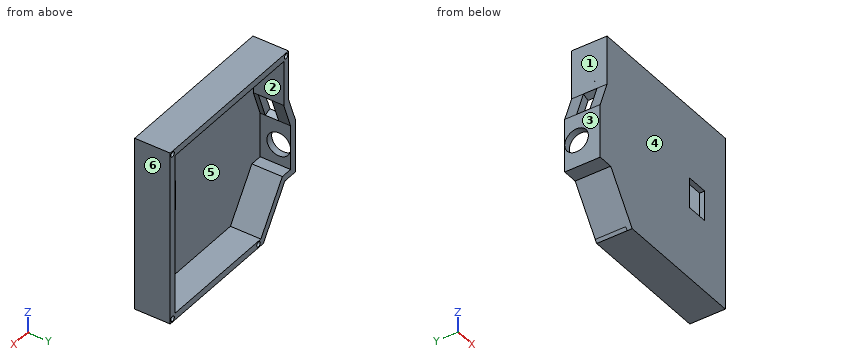
Autodesk Inventor part; units mm, degrees
ref_plane "YZ Plane" through (0, 0, 0) normal (1, 0, 0) x (0, 1, 0)
ref_plane "XZ Plane" through (0, 0, 0) normal (0, 1, 0) x (-1, 0, 0)
ref_plane "XY Plane" through (0, 0, 0) normal (0, 0, 1) x (1, 0, 0)
sketch "Sketch1" plane through (0, 0, 0) normal (0, 1, 0) x (-1, 0, 0)
  line L0 (0, 0) -> (49.1, 0)
  line L1 (49.1, -47.9) -> (0, -47.9)
  line L2 (0, -47.9) -> (0, 0)
  line L3 (46.7, -10.9) -> (49.1, -18.9)
  line L4 (46.7, -10.9) -> (46.7, 0)
  line L5 (49.1, 0) -> (46.7, 0)
  line L6 (49.1, -18.9) -> (49.1, -47.9)
  dimension "d0" = 49.1
  dimension "d1" = 47.9
  dimension "d2" = 18.9
extrude "Extrusion1" add sketch "Sketch1" along normal blind 1.5
sketch "Sketch2" plane through (0, 1.5, 0) normal (0, 1, 0) x (1, 0, 0)
  line L0 (-49.1, 18.9) -> (-46.7, 10.9)
  line L1 (-46.2, 10.9) -> (-46.2, 0)
  line L2 (-46.2, 0) -> (-46.7, 0)
  line L3 (-46.7, 10.9) -> (-46.7, 0)
  line L4 (-46.7, 0) -> (-46.7, 10.9)
  line L5 (-49.1, 47.9) -> (-49.1, 18.9)
  line L6 (-46.7, 10.9) -> (-49.1, 18.9)
  line L7 (-49.1, 18.9) -> (-46.2, 10.9)
  point P0 (0, 0)
extrude "Extrusion2" cut sketch "Sketch2" against normal blind 10
sketch "Sketch3" plane through (0, 1.5, 0) normal (0, 1, 0) x (1, 0, 0)
  line L0 (-49.1, 47.9) -> (-49.1, 18.9)
  line L1 (-49.1, 34.5784) -> (-45.5979, 34.5784)
  line L2 (-45.5979, 34.5784) -> (-36.4784, 47.9)
  line L3 (0, 47.9) -> (-49.1, 47.9)
  line L4 (-49.1, 47.9) -> (-36.4784, 47.9)
  line L5 (-49.1, 47.9) -> (-49.1, 34.5784)
  point P0 (0, 0)
extrude "Extrusion3" cut sketch "Sketch3" against normal blind 10
sketch "Sketch4" plane through (0, 1.5, 0) normal (0, 1, 0) x (1, 0, 0)
  line L0 (-46.2, 10.9) -> (-49.1, 18.9)
  line L1 (-46.2, 0) -> (0, 0)
  line L2 (-46.2, -2) -> (0, -2)
  line L3 (0, -2) -> (2, -2)
  line L4 (2, -2) -> (2, 47.9)
  line L5 (0, 47.9) -> (-36.4784, 47.9)
  line L6 (2, 47.9) -> (2, 49.9)
  line L7 (2, 49.9) -> (-36.4784, 49.9)
  line L8 (-38.1287, 49.0298) -> (-37.533, 49.9)
  line L9 (-37.533, 49.9) -> (-36.4784, 49.9)
  line L10 (-45.5979, 34.5784) -> (-36.4784, 47.9)
  line L11 (-49.1, 36.5784) -> (-46.6525, 36.5784)
  line L12 (-46.6525, 36.5784) -> (-37.533, 49.9)
  line L13 (-46.2, -2) -> (-48.2, -2)
  line L14 (-48.2, -2) -> (-48.2, 10.9)
  line L15 (-51.1, 18.9) -> (-48.2, 10.9)
  line L16 (-49.1, 36.5784) -> (-51.1, 36.5784)
  line L17 (-51.1, 36.5784) -> (-51.1, 18.9)
  line L18 (0, 0) -> (0, 47.9)
  line L19 (0, 0) -> (0, 47.9)
  line L20 (0, 47.9) -> (-36.4784, 47.9)
  line L21 (-36.4784, 47.9) -> (-45.5979, 34.5784)
  line L22 (-45.5979, 34.5784) -> (-49.1, 34.5784)
  line L23 (-49.1, 34.5784) -> (-45.5979, 34.5784)
  line L24 (-49.1, 34.5784) -> (-49.1, 18.9)
  line L25 (-49.1, 34.5784) -> (-49.1, 18.9)
  line L26 (-49.1, 18.9) -> (-46.2, 10.9)
  line L27 (-46.2, 0) -> (-46.2, 10.9)
  line L28 (-46.2, 0) -> (0, 0)
  dimension "d16" = 2
  dimension "d17" = 2
  dimension "d18" = 2
  dimension "d23" = 2
extrude "Extrusion4" add sketch "Sketch4" along normal blind 9
sketch "Sketch5" plane through (0, 0, 0) normal (0, -1, 0) x (1, 0, 0)
  line L0 (-46.2, 0) -> (0, 0)
  line L1 (0, 0) -> (-46.2, 0)
  line L2 (-46.2, 0) -> (-46.2, -10.9)
  line L3 (-46.2, 0) -> (-46.2, -10.9)
  line L4 (-46.2, -10.9) -> (-49.1, -18.9)
  line L5 (-46.2, -10.9) -> (-49.1, -18.9)
  line L6 (-49.1, -18.9) -> (-49.1, -34.5784)
  line L7 (-49.1, -18.9) -> (-49.1, -34.5784)
  line L8 (-49.1, -34.5784) -> (-45.5979, -34.5784)
  line L9 (-49.1, -34.5784) -> (-45.5979, -34.5784)
  line L10 (-36.4784, -47.9) -> (-45.5979, -34.5784)
  line L11 (-45.5979, -34.5784) -> (-36.4784, -47.9)
  line L12 (-36.4784, -47.9) -> (0, -47.9)
  line L13 (-36.4784, -47.9) -> (0, -47.9)
  line L14 (0, -47.9) -> (0, 0)
  line L15 (-48.2, 2) -> (2, 2)
  line L16 (2, 2) -> (-48.2, 2)
  line L17 (-51.1, -18.9) -> (-48.2, -10.9)
  line L18 (-48.2, 2) -> (-48.2, -10.9)
  line L19 (-48.2, -10.9) -> (-51.1, -18.9)
  line L20 (-51.1, -18.9) -> (-51.1, -36.5784)
  line L21 (-46.6525, -36.5784) -> (-51.1, -36.5784)
  line L22 (-51.1, -36.5784) -> (-46.6525, -36.5784)
  line L23 (-37.533, -49.9) -> (-46.6525, -36.5784)
  line L24 (-46.6525, -36.5784) -> (-37.533, -49.9)
  line L25 (2, 2) -> (2, -49.9)
  line L26 (-37.533, -49.9) -> (2, -49.9)
  line L27 (2, -49.9) -> (2, 2)
extrude "Extrusion5" add sketch "Sketch5" against normal blind 1.5
sketch "Sketch6" plane through (0, 10.5, 0) normal (0, 1, 0) x (1, 0, 0)
  line L0 (-48.2, -2) -> (2, -2)
  circle A0 centre (1, -1) radius 0.75
  line L1 (-46.2, 0) -> (-46.2, 10.9)
  circle A1 centre (-47.2, -1) radius 0.75
  point P0 (0, 0)
  dimension "d35" = 1.5
sketch "Sketch7" plane through (0, 10.5, 0) normal (0, 1, 0) x (1, 0, 0)
  point P0 (0, 0)
extrude "Extrusion6" cut sketch "Sketch6" against normal blind 7.5
sketch "Sketch8" plane through (0, 10.5, 0) normal (0, 1, 0) x (1, 0, 0)
  line L0 (-45.5979, 34.5784) -> (-36.4784, 47.9)
  circle A0 centre (-35.4784, 48.9) radius 0.75
  circle A1 centre (1, 48.9) radius 0.75
  point P0 (0, 0)
  dimension "d40" = 1.5
  dimension "d43" = 1.5
extrude "Extrusion7" cut sketch "Sketch8" against normal blind 7.5
sketch "Sketch9" plane through (0, 0, 0) normal (0, -1, 0) x (1, 0, 0)
  line L0 (-48.2, 2) -> (2, 2)
  line L1 (2, 2) -> (2, -49.9)
  line L2 (-6.75, -23.95) -> (-6.75, -19.45)
  line L3 (-6.75, -19.45) -> (-13.25, -19.45)
  line L4 (-13.25, -19.45) -> (-13.25, -28.45)
  line L5 (-13.25, -28.45) -> (-6.75, -28.45)
  line L6 (-6.75, -28.45) -> (-6.75, -23.95)
  point P0 (0, 0)
  dimension "d51" = 6.5
  dimension "d52" = 9
extrude "Extrusion8" cut sketch "Sketch9" against normal blind 1.5
sketch "Sketch10" plane through (0, 10.5, 0) normal (0, 1, 0) x (1, 0, 0)
  line L0 (-49.1, 18.9) -> (-46.2, 10.9)
  line L1 (-48.2, -2) -> (-48.2, 10.9)
  line L2 (-48.2, 10.9) -> (-51.1, 18.9)
  line L3 (-48.2, 10.175) -> (-48.2, 10.9)
  line L4 (-51.1, 18.9) -> (-51.1, 36.5784)
  line L5 (-51.1, 18.175) -> (-51.1, 18.9)
  line L6 (-51.1, 18.175) -> (-48.2, 10.175)
  line L7 (-48.2, 10.9) -> (-51.1, 18.9)
  point P0 (0, 0)
extrude "Extrusion9" add sketch "Sketch10" against normal blind 10.5
sketch "Sketch11" plane through (-51.1, 0, -18.175) normal (-0.9401361, 0, 0.3407993) x (0.3407993, 0, 0.9401361)
  point P0 (34.5018, 0)
sketch "Sketch12" plane through (-51.1, 0, -18.175) normal (-0.9401361, 0, 0.3407993) x (0.3407993, 0, 0.9401361)
  line L0 (0, 10.5) -> (0, 0)
  line L1 (5.4546, 0) -> (3.2394, 0)
  line L2 (4.2545, 0) -> (7.2545, 0) construction
  line L3 (4.2545, 7) -> (0, 7)
  line L4 (0, 7) -> (0, 3)
  line L5 (0, 3) -> (8.5094, 3)
  line L6 (8.5094, 1.5) -> (8.5094, 10.5)
  line L7 (4.2545, 7) -> (8.5094, 7)
  line L8 (8.5094, 10.5) -> (8.5094, 0)
  line L9 (8.5094, 3) -> (8.5094, 7)
  line L10 (0, 10.5) -> (8.5094, 10.5)
  line L11 (0, 10.5) -> (0, 0)
  line L12 (8.5094, 0) -> (0, 0)
  line L13 (8.5094, 10.5) -> (8.5094, 0)
  point P0 (34.5018, 0)
  dimension "d58" = 4.2545
extrude "Extrusion10" cut sketch "Sketch12" along normal blind 5 contours L3 L7 L6 L5 L0
sketch "Sketch14" plane through (0, 10.5, 0) normal (0, 1, 0) x (1, 0, 0)
  point P0 (0, 0)
sketch "Sketch15" plane through (0, 10.5, 0) normal (0, 1, 0) x (1, 0, 0)
  line L0 (-46.2, 0) -> (-46.2, 10.9)
  line L1 (-46.2, 10.9) -> (-46.2, 11.9)
  line L2 (-46.2, 11.9) -> (-49.1, 19.8981)
  line L3 (-49.1, 34.5784) -> (-49.1, 18.9)
  line L4 (-46.2, 11.9) -> (-37.6924, 11.9) construction
  line L5 (-49.1, 19.8981) -> (-49.1, 18.9)
  line L6 (-49.1, 18.9) -> (-46.2, 10.9)
  line L7 (-49.1, 18.9) -> (-46.2, 10.9)
  point P0 (0, 0)
  dimension "d71" = 1
  dimension "d72" = 109.93
extrude "Extrusion12" add sketch "Sketch15" against normal blind 9
sketch "Sketch16" plane through (0, 10.5, 0) normal (0, 1, 0) x (1, 0, 0)
  line L0 (-51.1, 18.175) -> (-48.2, 10.175)
  line L1 (-51.1, 18.175) -> (-51.1, 19.175)
  line L2 (-51.1, 36.5784) -> (-51.1, 18.175)
  line L3 (-51.1, 19.175) -> (-48.2, 11.1769)
  line L4 (-51.1, 19.175) -> (-42.5924, 19.175) construction
  line L5 (-48.2, 11.1769) -> (-48.2, 10.175)
  line L6 (-48.2, 10.175) -> (-48.2, -2)
  line L7 (-51.1, 18.175) -> (-48.2, 10.175)
  point P0 (0, 0)
  dimension "d75" = 1
  dimension "d76" = 70.07
extrude "Extrusion13" cut sketch "Sketch16" against normal blind 10.5
sketch "Sketch17" plane through (-51.1, 0, -36.5784) normal (-1, 0, 0) x (0, 0, 1)
  line L0 (-13.3216, 0) -> (-13.3216, 10.5)
  line L1 (36.8284, 10.5) -> (36.8284, 3)
  line L2 (38.5784, 0) -> (38.5784, 10.5)
  line L3 (15.9784, 5.25) -> (15.9784, 10.5) construction
  line L4 (16.6804, 10.5) -> (2, 10.5)
  point P0 (36.5784, 0)
sketch "Sketch18" plane through (0, 10.5, 0) normal (0, 1, 0) x (1, 0, 0)
  line L0 (-51.1, 19.175) -> (-51.1, 36.5784)
  line L1 (-51.1, 19.175) -> (-51.1, 20.6)
  line L2 (-51.1, 20.6) -> (-48.2, 12.6019)
  line L3 (-51.1, 20.6) -> (-42.5924, 20.6) construction
  line L4 (-51.1, 19.175) -> (-48.2, 11.1769)
  line L5 (-48.2, 12.6019) -> (-48.2, 11.1769)
  line L6 (-51.1, 19.175) -> (-48.2, 11.1769)
  point P0 (0, 0)
  dimension "d82" = 1.425
  dimension "d83" = 70.07
extrude "Extrusion14" cut sketch "Sketch18" against normal blind 10.5
sketch "Sketch19" plane through (0, 10.5, 0) normal (0, 1, 0) x (1, 0, 0)
  line L0 (-46.2, 11.9) -> (-49.1, 19.8981)
  line L1 (-46.2, 11.9) -> (-46.2, 13.325)
  line L2 (-46.2, 13.325) -> (-49.1, 21.3231)
  line L3 (-49.1, 19.8981) -> (-49.1, 34.5784)
  line L4 (-49.1, 21.3231) -> (-49.1, 19.8981)
  line L5 (-49.1, 19.8981) -> (-46.2, 11.9)
  point P0 (0, 0)
  dimension "d86" = 1.425
  dimension "d87" = 160.07
extrude "Extrusion15" add sketch "Sketch19" against normal blind 9
sketch "Sketch20" plane through (-51.1, 0, -20.6) normal (-0.9401098, 0, 0.3408718) x (0.3408718, 0, 0.9401098)
  line L0 (0, 3) -> (8.5096, 3)
  line L1 (8.5096, 10.5) -> (8.5096, 1.5)
  line L2 (8.5096, 3) -> (8.5096, 7)
  line L3 (8.5096, 7) -> (0.002, 7)
  line L4 (0.002, 10.5) -> (0.002, 1.5)
  line L5 (0, 3) -> (0.002, 7)
  point P0 (36.7848, 0)
  point P1 (0, 0)
  point P2 (8.5096, 7)
  dimension "d90" = 3
  dimension "d91" = 4
extrude "Extrusion16" cut sketch "Sketch20" against normal blind 10
sketch "Sketch21" plane through (-51.1, 0, -36.5784) normal (-1, 0, 0) x (0, 0, 1)
  point P0 (36.5784, 0)
sketch "Sketch22" plane through (-51.1, 0, -36.5784) normal (-1, 0, 0) x (0, 0, 1)
  line L0 (15.9784, 0) -> (0, 0)
  line L1 (17.1284, 0) -> (8.1284, 0)
  circle A0 centre (8.1284, 7) radius 3.5
  point P0 (36.5784, 0)
  dimension "d98" = 7
extrude "Extrusion17" cut sketch "Sketch22" against normal blind 10
properties part number "Case"
The model under review builds one solid part; all positions refer to its coordinate system, in mm. Face numbers are marked on the shaded views. A direction names the side the tool comes from. Coordinates: 2 decimals unless noted, no trailing zeros. Write each loop counter-clockwise with the first axis right and the second up, starting at its lowest first coordinate (ties: lowest second). Pieces come first, ordered by that corner, then holes.
1) Machinability: for the marked faces 1, 2 and 3, which of the approach directions +Z, -Z, +X, -X, +Y, -Y give a long, thin tool a straight path to every point of the face, cutting with its end or side? Answer none if there is none.
2) We need section B-B on y = 2.25. State the section outline as (x, z) points (1 decimal), then the cut area to 3 significant figures.
3) We need section C-C on z = -1.5. State the section outline as (x, y) points.
4) Clearance check with flat-ended pins moving along their axes: pin 1 Ø1 at (x, z) = (-30.5, -19) entering from +Y; pin 2 Ø5 at (y, z) = (3.5, -2) entering from -X. State where each tip first meets the part, or that it passes through.
5) The part is to be moulded in two halves that separate along X. For the marked faces 4, 5 and 6, say which applies: pulls with the +X half, pulls with the -X half, needs draft (parallel to the pull), parting line crosses it, or undercut.
6) We need section D-D on y = 8.5. Count the separate pieces of the cut face and the enclosed holes in it, then the cut area to 3 significant figures.
7) To check wall thickness, follow probe 1 along Z at (x, y) = (1, 5.75); probe 2 along X at (y, z) = (8, 1); probe 3 along X at (y, z) = (5.75, -32.5). State the ranges of each line that lie inside material, in increasing order.
8) We need section A-A on x = -9. State the section outline as (y, z) points.
Answer list:
1. face 1: +Z, -X, +Y, -Y
1. face 2: +Y
1. face 3: +Z, -Z, -X, +Y, -Y
2. outline: (-51.1, -36.6) - (-46.7, -36.6) - (-38.1, -49) - (-37.5, -49.9) - (2, -49.9) - (2, 2) - (-48.2, 2) - (-48.2, -12.6) - (-51.1, -20.6) - close; hole (-49.1, -34.6) - (-45.6, -34.6) - (-36.5, -47.9) - (0, -47.9) - (0, 0) - (-46.2, 0) - (-46.2, -13.3) - (-49.1, -21.3) - close
2. area: 388 mm2
3. outline: (-48.2, 0) - (2, 0) - (2, 10.5) - (0, 10.5) - (0, 1.5) - (-46.2, 1.5) - (-46.2, 10.5) - (-48.2, 10.5) - close
4. pin 1: stops at y = 1.5
4. pin 2: stops at x = -48.2
5. face 4: needs draft
5. face 5: undercut
5. face 6: pulls with the +X half
6. separate pieces: 1
6. enclosed holes: 4
6. area: 368 mm2
7. probe 1: z = -49.9 to -49.65, -48.15 to 0.25, 1.75 to 2
7. probe 2: x = -48.2 to -47.95, -46.45 to 0.25, 1.75 to 2
7. probe 3: x = -51.1 to -49.1, 0 to 2
8. outline: (0, -49.9) - (10.5, -49.9) - (10.5, -47.9) - (1.5, -47.9) - (1.5, -28.45) - (0, -28.45) - close; (0, -19.45) - (1.5, -19.45) - (1.5, 0) - (10.5, 0) - (10.5, 2) - (0, 2) - close
